```python
from build123d import *

# Parameters (mm, degrees)
SKETCH1_W           = 203.2
SKETCH1_H           = 101.6
BOSS_EXTRUDE1_DEPTH = 6.35
SKETCH3_W           = 6.35
SKETCH3_H           = 12.7
CUT_EXTRUDE2_DEPTH  = 6.35
SKETCH4_W           = 6.35
SKETCH4_H           = 6.35
CUT_EXTRUDE3_DEPTH  = 6.35
LPATTERN1_COUNT     = 15
LPATTERN1_PITCH     = 12.7
SKETCH5_W           = 6.35
SKETCH5_H           = 6.35
CUT_EXTRUDE4_DEPTH  = 6.35
LPATTERN2_COUNT     = 7
LPATTERN2_PITCH     = 12.7
SKETCH6_W           = 6.35
SKETCH6_H           = 6.35
CUT_EXTRUDE5_DEPTH  = 6.35
SKETCH8_W           = 6.35
SKETCH8_H           = 6.35
CUT_EXTRUDE6_DEPTH  = 6.35
LPATTERN3_COUNT     = 7
LPATTERN3_PITCH     = 12.7
SKETCH9_R           = 3.96875
CUT_EXTRUDE7_DEPTH  = 6.35


with BuildPart() as part:
    # Sketch1 → Boss-Extrude1 (new body)
    with BuildSketch(Plane(origin=(0, 0, 0), x_dir=(0, 0, -1), z_dir=(1, 0, 0))):
        with Locations((101.6, 50.8)):
            Rectangle(SKETCH1_W, SKETCH1_H)
    extrude(amount=BOSS_EXTRUDE1_DEPTH)

    # Sketch3 → Cut-Extrude2 (cut)
    with BuildSketch(Plane.XZ):
        with Locations((3.175, -6.35)):
            Rectangle(SKETCH3_W, SKETCH3_H)
    extrude(amount=-CUT_EXTRUDE2_DEPTH, mode=Mode.SUBTRACT)

    # Sketch4 → Cut-Extrude3 (cut)
    with BuildSketch(Plane.XZ):
        with Locations((3.175, -22.225)):
            Rectangle(SKETCH4_W, SKETCH4_H)
    cut_extrude3 = extrude(amount=-CUT_EXTRUDE3_DEPTH, mode=Mode.SUBTRACT)

    # LPattern1: Cut-Extrude3 ×15
    with Locations(*[(0, 0, -i * LPATTERN1_PITCH) for i in range(1, LPATTERN1_COUNT)]):
        add(cut_extrude3, mode=Mode.SUBTRACT)

    # Sketch5 → Cut-Extrude4 (cut)
    with BuildSketch(Plane.XY):
        with Locations((3.175, 15.875)):
            Rectangle(SKETCH5_W, SKETCH5_H)
    cut_extrude4 = extrude(amount=-CUT_EXTRUDE4_DEPTH, mode=Mode.SUBTRACT)

    # LPattern2: Cut-Extrude4 ×7
    with Locations(*[(0, i * LPATTERN2_PITCH, 0) for i in range(1, LPATTERN2_COUNT)]):
        add(cut_extrude4, mode=Mode.SUBTRACT)

    # Sketch6 → Cut-Extrude5 (cut)
    with BuildSketch(Plane(origin=(0, 0, -203.2), x_dir=(-1, 0, 0), z_dir=(0, 0, -1))):
        with Locations((-3.175, 9.525)):
            Rectangle(SKETCH6_W, SKETCH6_H)
    extrude(amount=-CUT_EXTRUDE5_DEPTH, mode=Mode.SUBTRACT)

    # Sketch8 → Cut-Extrude6 (cut)
    with BuildSketch(Plane(origin=(0, 0, -203.2), x_dir=(-1, 0, 0), z_dir=(0, 0, -1))):
        with Locations((-3.175, 22.225)):
            Rectangle(SKETCH8_W, SKETCH8_H)
    cut_extrude6 = extrude(amount=-CUT_EXTRUDE6_DEPTH, mode=Mode.SUBTRACT)

    # LPattern3: Cut-Extrude6 ×7
    with Locations(*[(0, i * LPATTERN3_PITCH, 0) for i in range(1, LPATTERN3_COUNT)]):
        add(cut_extrude6, mode=Mode.SUBTRACT)

    # Sketch9 → Cut-Extrude7 (cut)
    with BuildSketch(Plane.ZY):
        with Locations((-171.45, 31.75)):
            Circle(SKETCH9_R)
    extrude(amount=-CUT_EXTRUDE7_DEPTH, mode=Mode.SUBTRACT)


solid = part.part
```
Can you work these out from the model? Positions are in its coordinate system, mm. A direction names the side the tool comes from. Round coordinates to 2 decimals unless told otherwise and drop trailing zeros. Answer as a JSON object with one key per item and string values. Group by question number.
Q1. We'd pull the mould along Z, two halves only. Please class faces 1 (the flat face through (3, 16, -6.35)), 2 (the flat face through (3, 6.35, -98)), 3 (the flat face through (3, 95.25, -3)): +Z half, -Z half, draft (parallel to the pull), parting line (faces both ways), or undercut.
Q2. On a 3-axis mill with a long thin cutter (end or side, diameter ignored), from which of +Z, -Z, +X, -X, +Y, -Y can I reach the whole of each face in a straight line? I mean faces 4 (the flat face through (3, 50.8, -3)), 5 (the flat face through (3, 98, 0)), 6 (the flat face through (3, 0, -168)), 7 (the flat face through (3, 98, -196.85)), 8 (the flat face through (3, 3, -165.1)). Say none if no direction works.
Q3. Will these pins go through, and if not, where does the flat tip stop? pin 1 (1.9 mm diameter, centred on x = 3.5, z = -200, fed in from -Y); pin 2 (3 mm diameter, centred on x = 4.5, z = -199, fed in from +Y); pin 3 (1.9 mm diameter, centred on x = 3.5, y = 3, fed in from +Z).
Q4. Please list where these lines run through material, in increasing order: L1, parallel to Y at x = 5.75, z = -161; L2, parallel to Z at x = 3.75, y = 80; L3, parallel to Z at x = 5.25, y = 48.
Findings:
{
 "1": {"face 1": "+Z half", "face 2": "undercut", "face 3": "draft"},
 "2": {"face 4": "+Z, +X, -X", "face 5": "+Z, +X, -X, +Y, -Y", "face 6": "+Z, -Z, +X, -X, -Y", "face 7": "-Z, +X, -X, +Y", "face 8": "+X, -X, -Y"},
 "3": {"pin 1": "stops at y = 12.7", "pin 2": "stops at y = 95.25", "pin 3": "stops at z = -12.7"},
 "4": {"L1": "y = 6.35 to 101.6", "L2": "z = -203.2 to -6.35", "L3": "z = -196.85 to 0"}
}
